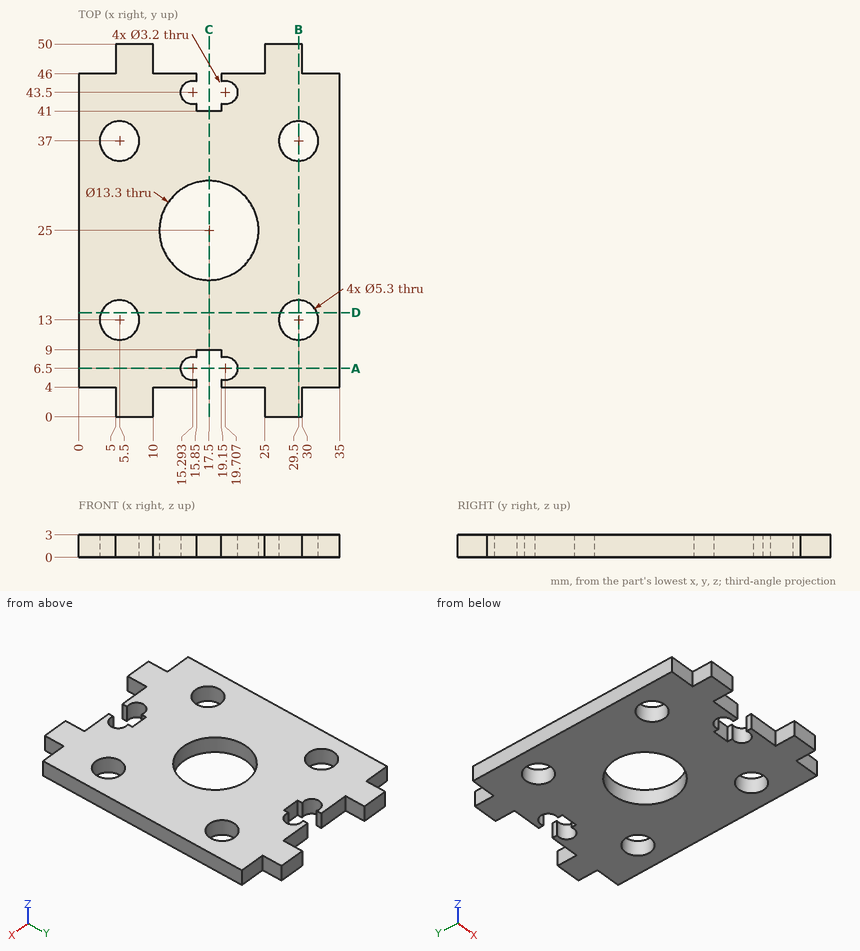
Answer from the drawing. Dimensions are ordinates in mm from the lowest x, y and z of the part. Coordinates: 2 decimals unless noted, no trailing zeros. Loops run counter-clockwise (first coordinate to the right, second up) from the corner with the lowest first, then second, coordinate; pieces in that order, holes last. Notation, with made-up numbers: (72, 29.5) -> (87, 29.5) arc R4 cw to (87, 35.5) -> close; hole circle Ø2 at (33, 40). An arc over 180 degrees is marked (long way). Answer as CSV lines item,"result".
Q1. The part is cut by section A-A on y = 6.5. Write down the section's boundary in (x, z).
Findings:
outline,"(0, 0) -> (13.69, 0) -> (13.69, 3) -> (0, 3) -> close; (21.31, 0) -> (35, 0) -> (35, 3) -> (21.31, 3) -> close"
Q2. The part is cut by section B-B on x = 29.5. Write down the section's boundary in (y, z).
Findings:
outline,"(0, 0) -> (10.35, 0) -> (10.35, 3) -> (0, 3) -> close; (15.65, 0) -> (34.35, 0) -> (34.35, 3) -> (15.65, 3) -> close; (39.65, 0) -> (50, 0) -> (50, 3) -> (39.65, 3) -> close"
Q3. The part is cut by section D-D on y = 14. Write down the section's boundary in (x, z) (1 decimal).
Findings:
outline,"(0, 0) -> (3, 0) -> (3, 3) -> (0, 3) -> close; (8, 0) -> (27, 0) -> (27, 3) -> (8, 3) -> close; (32, 0) -> (35, 0) -> (35, 3) -> (32, 3) -> close"
Q4. Each of these flat-tipped pins is pushed along its axis until it touches: pin 1 (5 mm diameter, centred on x = 15.29, y = 43.5, fed in from +Z); pin 2 (1.5 mm diameter, centred on y = 47.5, z = 2, fed in from +X); pin 3 (0.9 mm diameter, centred on x = 17, z = 2, fed in from +Y). Where does it stop, or does it pass through?
Findings:
pin 1,"stops at z = 3"
pin 2,"stops at x = 30"
pin 3,"stops at y = 41"
Q5. The part is cut by section C-C on x = 17.5. Write down the section's boundary in (y, z), and give its area (3 significant figures).
Findings:
outline,"(9, 0) -> (18.35, 0) -> (18.35, 3) -> (9, 3) -> close; (31.65, 0) -> (41, 0) -> (41, 3) -> (31.65, 3) -> close"
area,"56.1 mm²"
Q6. Find the intervals of material crossed by probe 1 along X at (y, z) = (3.5, 0.6); probe 2 along X at (y, z) = (6.5, 1.15); probe 3 along Y at (x, z) = (28.5, 0.35) (1 decimal), in increasing order.
Findings:
probe 1,"x = 5 to 10, 25 to 30"
probe 2,"x = 0 to 13.69, 21.31 to 35"
probe 3,"y = 0 to 10.5, 15.5 to 34.5, 39.5 to 50"
